from build123d import *

# Parameters (mm, degrees)
SKETCH1_R           = 46.5
SKETCH1_R_2         = 2.5
SKETCH1_R_3         = 17.5
BOSS_EXTRUDE1_DEPTH = 12.7
SKETCH2_R           = 28
CUT_EXTRUDE1_DEPTH  = 6.35
SKETCH3_R           = 2.5
CUT_EXTRUDE2_DEPTH  = 6.35
SKETCH4_R           = 3.25
CUT_EXTRUDE3_DEPTH  = 6.35


with BuildPart() as part:
    # Sketch1 → Boss-Extrude1 (new body)
    with BuildSketch(Plane(origin=(0, 0, 0), x_dir=(1, 0, 0), z_dir=(0, 1, 0))):
        with Locations(Location((0, 0, 0), (0, 0, 270))):
            Circle(SKETCH1_R)
        with Locations(Location((0, 32.5, 0), (0, 0, 270))):
            Circle(SKETCH1_R_2, mode=Mode.SUBTRACT)
        with Locations(Location((28.145825623, -16.25, 0), (0, 0, 270))):
            Circle(SKETCH1_R_2, mode=Mode.SUBTRACT)
        with Locations(Location((-28.145825623, -16.25, 0), (0, 0, 270))):
            Circle(SKETCH1_R_2, mode=Mode.SUBTRACT)
        with Locations(Location((0, 0, 0), (0, 0, 270))):
            Circle(SKETCH1_R_3, mode=Mode.SUBTRACT)
    extrude(amount=BOSS_EXTRUDE1_DEPTH)

    # Sketch2 → Cut-Extrude1 (cut)
    with BuildSketch(Plane(origin=(0, 12.7, 0), x_dir=(1, 0, 0), z_dir=(0, 1, 0))):
        with Locations(Location((0, 0, 0), (0, 0, 270))):
            Circle(SKETCH2_R)
    extrude(amount=-CUT_EXTRUDE1_DEPTH, mode=Mode.SUBTRACT)

    # Sketch3 → Cut-Extrude2 (cut)
    with BuildSketch(Plane(origin=(0, 12.7, 0), x_dir=(1, 0, 0), z_dir=(0, 1, 0))):
        with Locations(Location((0, 41, 0), (0, 0, 270))):
            Circle(SKETCH3_R)
        with Locations(Location((28.991378029, 28.991378029, 0), (0, 0, 270))):
            Circle(SKETCH3_R)
        with Locations(Location((41, 0, 0), (0, 0, 270))):
            Circle(SKETCH3_R)
        with Locations(Location((28.991378029, -28.991378029, 0), (0, 0, 270))):
            Circle(SKETCH3_R)
        with Locations(Location((0, -41, 0), (0, 0, 270))):
            Circle(SKETCH3_R)
        with Locations(Location((-28.991378029, -28.991378029, 0), (0, 0, 270))):
            Circle(SKETCH3_R)
        with Locations(Location((-41, 0, 0), (0, 0, 270))):
            Circle(SKETCH3_R)
        with Locations(Location((-28.991378029, 28.991378029, 0), (0, 0, 270))):
            Circle(SKETCH3_R)
    extrude(amount=-CUT_EXTRUDE2_DEPTH, mode=Mode.SUBTRACT)

    # Sketch4 → Cut-Extrude3 (cut)
    with BuildSketch(Plane(origin=(0, 12.7, 0), x_dir=(1, 0, 0), z_dir=(0, 1, 0))):
        with Locations(Location((0, 32.5, 0), (0, 0, 270))):
            Circle(SKETCH4_R)
        with Locations(Location((28.145825623, -16.25, 0), (0, 0, 270))):
            Circle(SKETCH4_R)
        with Locations(Location((-28.145825623, -16.25, 0), (0, 0, 270))):
            Circle(SKETCH4_R)
        Polygon((0, 45.618802154), (-4, 43.309401077), (-4, 38.690598923), (0, 36.381197846), (4, 38.690598923), (4, 43.309401077), align=None)
        Polygon((33.452798315, 27.795944066), (32.257364352, 32.257364352), (27.795944066, 33.452798315), (24.529957742, 30.186811992), (25.725391705, 25.725391705), (30.186811992, 24.529957742), align=None)
        Polygon((43.309401077, -4), (45.618802154, 0), (43.309401077, 4), (38.690598923, 4), (36.381197846, 0), (38.690598923, -4), align=None)
        Polygon((27.795944066, -33.452798315), (32.257364352, -32.257364352), (33.452798315, -27.795944066), (30.186811992, -24.529957742), (25.725391705, -25.725391705), (24.529957742, -30.186811992), align=None)
        Polygon((-4, -43.309401077), (0, -45.618802154), (4, -43.309401077), (4, -38.690598923), (0, -36.381197846), (-4, -38.690598923), align=None)
        Polygon((-33.452798315, -27.795944066), (-32.257364352, -32.257364352), (-27.795944066, -33.452798315), (-24.529957742, -30.186811992), (-25.725391705, -25.725391705), (-30.186811992, -24.529957742), align=None)
        Polygon((-43.309401077, 4), (-45.618802154, 0), (-43.309401077, -4), (-38.690598923, -4), (-36.381197846, 0), (-38.690598923, 4), align=None)
        Polygon((-27.795944066, 33.452798315), (-32.257364352, 32.257364352), (-33.452798315, 27.795944066), (-30.186811992, 24.529957742), (-25.725391705, 25.725391705), (-24.529957742, 30.186811992), align=None)
    extrude(amount=-CUT_EXTRUDE3_DEPTH, mode=Mode.SUBTRACT)


solid = part.part
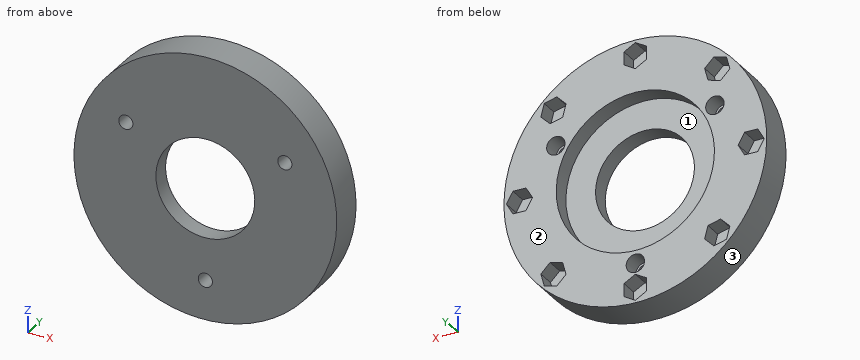
Part model, mm, in its own coordinate system. Face numbers are marked on the shaded views. Give positions to 0.01 mm unless a question says otherwise; leave off trailing zeros. Order: outer loops, then holes, each group sorted by start corner. A loop starts at its lowest first (then second) coordinate and runs counter-clockwise, first axis right, second up. Notation, with made-up numbers: (-8, 44) - (0, 44) arc R27 cw to (0, 69) - close; hole circle Ø2 at (-25, 69.25). An arc over 180 degrees is marked (long way). Use a Markdown table: item, result.
1) Probe L1, parallel to X at y = 10, z = 0; L2, parallel to X at y = 4.75, z = 0; L3, parallel to X at y = 8.25, z = 16.25. List the from-to ranges inside material, lowest first. Write a range as from..to.
Checked values:
| item | result |
|---|---|
| L1 | -46.5..-45.62, -36.38..-28, 28..36.38, 45.62..46.5 |
| L2 | -46.5..-17.5, 17.5..46.5 |
| L3 | -43.57..-31.4, -24.9..-22.8, 22.8..24.9, 31.4..43.57 |
2) Saw through at A-A on x = 6.5. List the corners of the cut face in (y, z).
Checked values:
| item | result |
|---|---|
| outline | (0, -46.04) - (12.7, -46.04) - (12.7, -27.24) - (6.35, -27.24) - (6.35, -16.25) - (0, -16.25) - close; (0, 16.25) - (6.35, 16.25) - (6.35, 27.24) - (12.7, 27.24) - (12.7, 46.04) - (0, 46.04) - close |
3) Saw through at C-C on y = 5.25. List the corners of the cut face in (x, z).
Checked values:
| item | result |
|---|---|
| outline | circle Ø93 at (0, 0); hole circle Ø5 at (-28.15, 16.25); hole circle Ø35 at (0, 0); hole circle Ø5 at (0, -32.5); hole circle Ø5 at (28.15, 16.25) |
4) Saw through at D-D on x = -14.5. List the corners of the cut face in (y, z).
Checked values:
| item | result |
|---|---|
| outline | (0, -44.18) - (12.7, -44.18) - (12.7, -23.95) - (6.35, -23.95) - (6.35, -9.8) - (0, -9.8) - close; (0, 9.8) - (6.35, 9.8) - (6.35, 23.95) - (12.7, 23.95) - (12.7, 44.18) - (0, 44.18) - close |
5) Flat gauge pins, fed straight in: P1, Ø1.4, axis at y = 10.5, z = 40.5, coming from the +X side; P2, Ø2.5, axis at x = 42, y = 9, coming from the -Z side; P3, Ø1.4, axis at x = -41.5, y = 10.5, coming from the +Z side; P4, Ø4, axis at x = 0, z = -32.5, coming from the -Y side. Where does each tip first touch, or does it go through?
Checked values:
| item | result |
|---|---|
| P1 | x = 24.05 |
| P2 | z = -22.4 |
| P3 | z = 22.31 |
| P4 | through |
6) Two-plate mould, pull along X, no slides. Class the marked faces 1, 2 and 3: +X half, -X half, draft (parallel to the pull), parting line (faces both ways), or undercut.
Checked values:
| item | result |
|---|---|
| face 1 | undercut |
| face 2 | draft |
| face 3 | parting line |
7) Saw through at B-B on z = -21.5. List the corners of the cut face in (x, y), plus the area to 3 significant figures.
Checked values:
| item | result |
|---|---|
| outline | (-41.23, 0) - (41.23, 0) - (41.23, 12.7) - (17.94, 12.7) - (17.94, 6.35) - (-17.94, 6.35) - (-17.94, 12.7) - (-41.23, 12.7) - close |
| area | 819 mm² |
